For this review, take the finished solid that the model builds, in its own axes (mm). Round coordinates to 2 decimals unless told otherwise and drop trailing zeros. Order: outer loops, then holes, each group sorted by start corner. A loop starts at its lowest first (then second) coordinate and runs counter-clockwise, first axis right, second up. Notation, with made-up numbers: M 1.5,-22 L 18.5,-22 A18 ccw 18.5,-13 Z; hole C 77.25,17 d6. An arc over 180 degrees is marked long. Use a Markdown table: item, result.
Autodesk Inventor part; units mm, degrees
ref_plane "YZ Plane" through (0, 0, 0) normal (1, 0, 0) x (0, 1, 0)
ref_plane "XZ Plane" through (0, 0, 0) normal (0, 1, 0) x (-1, 0, 0)
ref_plane "XY Plane" through (0, 0, 0) normal (0, 0, 1) x (1, 0, 0)
sketch "Sketch1" plane through (0, 0, 0) normal (0, 0, 1) x (1, 0, 0)
  line L0 (0, 0) -> (0, 38.1)
  line L1 (0, 38.1) -> (128.1684, 38.1)
  line L2 (128.1684, 38.1) -> (128.1684, 0)
  line L3 (128.1684, 0) -> (0, 0)
  dimension "d0" = 38.1
  dimension "d1" = 128.1684
extrude "Extrusion1" add sketch "Sketch1" along normal blind 3.175
sketch "Sketch2" plane through (0, 0, 3.175) normal (0, 0, 1) x (1, 0, 0)
  line L0 (128.1684, 38.1) -> (0, 38.1)
  line L1 (0, 38.1) -> (12.7, 38.1)
  line L2 (12.7, 38.1) -> (12.7, 31.75)
  line L3 (12.7, 31.75) -> (12.7, 6.35)
  circle A0 centre (12.7, 31.75) radius 3.3782
  circle A1 centre (12.7, 6.35) radius 3.3782
  line L4 (128.1684, 38.1) -> (115.4684, 38.1)
  line L5 (115.4684, 38.1) -> (115.4684, 31.75)
  circle A2 centre (115.4684, 31.75) radius 3.3782
  circle A3 centre (115.4684, 6.35) radius 3.3782
  line L6 (115.4684, 6.35) -> (115.4684, 31.75)
  dimension "d4" = 12.7
  dimension "d5" = 6.35
  dimension "d6" = 25.4
  dimension "d7" = 6.7564
  dimension "d8" = 6.7564
  dimension "d9" = 12.7
  dimension "d10" = 6.35
  dimension "d11" = 6.7564
  dimension "d12" = 6.7564
  dimension "d13" = 25.4
extrude "Extrusion2" cut sketch "Sketch2" against normal blind 3.175
fillet "Fillet1" radius 3.175 4 edges at (128.1684, 38.1, 1.5875) (128.1684, 0, 1.5875) (0, 38.1, 1.5875) (0, 0, 1.5875)
sketch "Sketch3" plane through (0, 0, 3.175) normal (0, 0, 1) x (1, 0, 0)
  arc A0 (0, 3.175) -> (3.175, 0) centre (3.175, 3.175) ccw
  line L0 (3.175, 0) -> (124.9934, 0)
  arc A1 (124.9934, 0) -> (128.1684, 3.175) centre (124.9934, 3.175) ccw
  line L1 (128.1684, 3.175) -> (128.1684, 34.925)
  arc A2 (128.1684, 34.925) -> (124.9934, 38.1) centre (124.9934, 34.925) ccw
  line L2 (124.9934, 38.1) -> (3.175, 38.1)
  arc A3 (3.175, 38.1) -> (0, 34.925) centre (3.175, 34.925) ccw
  line L3 (0, 34.925) -> (0, 3.175)
  circle A4 centre (115.4684, 31.75) radius 3.3782
  circle A5 centre (12.7, 31.75) radius 3.3782
  circle A6 centre (12.7, 6.35) radius 3.3782
  circle A7 centre (115.4684, 6.35) radius 3.3782
  line L4 (128.1684, 38.1) -> (102.7684, 38.1)
  line L5 (102.7684, 38.1) -> (102.7684, 0)
  point P0 (0, 0)
  dimension "d17" = 25.4
properties part number "anti - chain tension" material "Aluminum 6061"
Q1. Add section A-A (y = 6.35). Write out the cut boundary in (x, z) (3 decimals), then the cut area to 3 significant figures.
Determined:
| item | result |
|---|---|
| outline | M 0,0 L 9.322,0 L 9.322,3.175 L 0,3.175 Z; M 16.078,0 L 112.09,0 L 112.09,3.175 L 16.078,3.175 Z; M 118.847,0 L 128.168,0 L 128.168,3.175 L 118.847,3.175 Z |
| area | 364 mm^2 |
Q2. Add section B-B (x = 12.7). Write out the cut boundary in (y, z) (3 decimals).
Determined:
| item | result |
|---|---|
| outline | M 0,0 L 2.972,0 L 2.972,3.175 L 0,3.175 Z; M 9.728,0 L 28.372,0 L 28.372,3.175 L 9.728,3.175 Z; M 35.128,0 L 38.1,0 L 38.1,3.175 L 35.128,3.175 Z |
Q3. Wall thickness on line 1 along Y through (x, z) = (12.7, 2.3); line 2 along X through (y, z) = (6.35, 1); line 3 along X through (y, z) = (29.5, 2.75): over which ranges is each line inside the solid? List them lowest first. Write a range as [from, to].
Determined:
| item | result |
|---|---|
| line 1 | y = [0, 2.97], [9.73, 28.37], [35.13, 38.1] |
| line 2 | x = [0, 9.32], [16.08, 112.09], [118.85, 128.17] |
| line 3 | x = [0, 10.18], [15.22, 112.95], [117.99, 128.17] |
Q4. Draft analysis for pull direction X (two halves, no side actions). For faces 1 (the cylindrical face through (127.26, 37.15, 1.61)), 2 (the cylindrical face through (112.093, 6.499, 1.61)), 3 (the flat face through (63, 38.1, 2)), 4 (the cylindrical face through (9.325, 6.499, 1.61)), state which applies: pulls with the +X half, pulls with the -X half, needs draft (parallel to the pull), parting line crosses it, or undercut.
Determined:
| item | result |
|---|---|
| face 1 | pulls with the +X half |
| face 2 | undercut |
| face 3 | needs draft |
| face 4 | undercut |
Q5. Add section C-C (z = 1.6). Write out the cut boundary in (x, y) (3 decimals), then the cut area to 3 significant figures.
Determined:
| item | result |
|---|---|
| outline | M 0,3.175 A3.175 ccw 3.175,0 L 124.993,0 A3.175 ccw 128.168,3.175 L 128.168,34.925 A3.175 ccw 124.993,38.1 L 3.175,38.1 A3.175 ccw 0,34.925 Z; hole C 12.7,6.35 d6.756; hole C 12.7,31.75 d6.756; hole C 115.468,6.35 d6.756; hole C 115.468,31.75 d6.756 |
| area | 4,730 mm^2 |
